Build history of the part. All positions in model axes, mm. Round coordinates to 2 decimals unless told otherwise and drop trailing zeros. Loops run counter-clockwise (first coordinate to the right, second up) from the corner with the lowest first, then second, coordinate; pieces in that order, holes last. Notation, with made-up numbers: (31, -35) - (76, -35) arc R25 cw to (76, -1) - close; hole circle Ø6 at (34.25, 53.5). An arc over 180 degrees is marked (long way). Use a Markdown table: item, result.
from build123d import *

# Parameters (mm, degrees)
SKETCH1_R           = 15
BOSS_EXTRUDE1_DEPTH = 3.175
SKETCH2_R           = 1.7
SKETCH2_R_2         = 2.65
CUT_EXTRUDE1_DEPTH  = 4.175
FILLET1_R           = 5


with BuildPart() as part:
    # Sketch1 → Boss-Extrude1 (new body)
    with BuildSketch(Plane.XY):
        Polygon((-22, 22), (22, 22), (38.014690308, -22), (38.014690308, -42), (-38.014690308, -42), (-38.014690308, -22), align=None)
        Circle(SKETCH1_R, mode=Mode.SUBTRACT)
    extrude(amount=BOSS_EXTRUDE1_DEPTH)

    # Sketch2 → Cut-Extrude1 (cut, through all)
    with BuildSketch(Plane.XY.offset(3.175)):
        with Locations((15.5, 15.5)):
            Circle(SKETCH2_R)
        with Locations((15.5, -15.5)):
            Circle(SKETCH2_R)
        with Locations((-15.5, -15.5)):
            Circle(SKETCH2_R)
        with Locations((-15.5, 15.5)):
            Circle(SKETCH2_R)
        with Locations((0, -32)):
            Circle(SKETCH2_R_2)
        with Locations((28.014690308, -32)):
            Circle(SKETCH2_R_2)
        with Locations((-28.014690308, -32)):
            Circle(SKETCH2_R_2)
    extrude(amount=-CUT_EXTRUDE1_DEPTH, mode=Mode.SUBTRACT)

    # Fillet1
    fillet1_edges = [part.edges().sort_by_distance(p)[0] for p in [
        (38.014690308, -22, 1.5875),
        (38.014690308, -42, 1.5875),
        (-38.014690308, -42, 1.5875),
        (-38.014690308, -22, 1.5875),
        (-22, 22, 1.5875),
        (22, 22, 1.5875),
    ]]
    fillet(fillet1_edges, radius=FILLET1_R)


solid = part.part
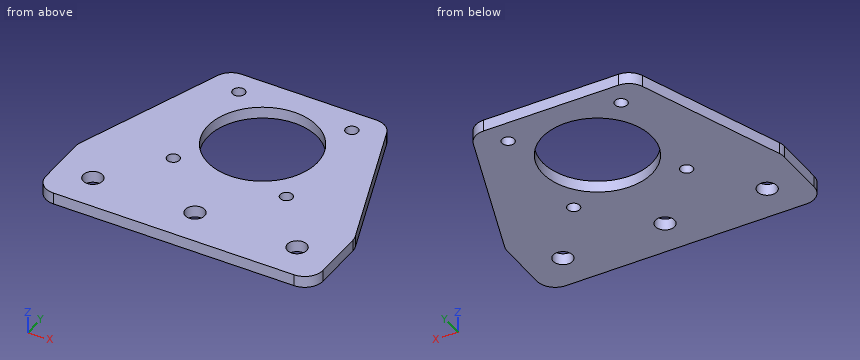
Q1. Cut at B-B, the plane y = -32. List the corners of the cut face in (x, z) (3 decimals), plus the area to 3 significant figures.
Results found:
| item | result |
|---|---|
| outline | (-38.015, 0) - (-30.665, 0) - (-30.665, 3.175) - (-38.015, 3.175) - close; (-25.365, 0) - (-2.65, 0) - (-2.65, 3.175) - (-25.365, 3.175) - close; (2.65, 0) - (25.365, 0) - (25.365, 3.175) - (2.65, 3.175) - close; (30.665, 0) - (38.015, 0) - (38.015, 3.175) - (30.665, 3.175) - close |
| area | 191 mm2 |
Q2. Cut at A-A, the plane x = -12. List the corners of the cut face in (y, z) (3 decimals).
Results found:
| item | result |
|---|---|
| outline | (-42, 0) - (-9, 0) - (-9, 3.175) - (-42, 3.175) - close; (9, 0) - (22, 0) - (22, 3.175) - (9, 3.175) - close |
Q3. Cut at C-C, the plane x = 0. List the corners of the cut face in (y, z) (3 decimals).
Results found:
| item | result |
|---|---|
| outline | (-42, 0) - (-34.65, 0) - (-34.65, 3.175) - (-42, 3.175) - close; (-29.35, 0) - (-15, 0) - (-15, 3.175) - (-29.35, 3.175) - close; (15, 0) - (22, 0) - (22, 3.175) - (15, 3.175) - close |
Q4. Probe line 1 (Y direction, x = -15.5, z = 0.7); line 2 (Y direction, x = 0, z = 1.05); line 3 (Y direction, x = -3, z = 0.5). List the from-to ranges inside material, lowest first.
Results found:
| item | result |
|---|---|
| line 1 | y = -42 to -17.2, -13.8 to 13.8, 17.2 to 22 |
| line 2 | y = -42 to -34.65, -29.35 to -15, 15 to 22 |
| line 3 | y = -42 to -14.7, 14.7 to 22 |
Q5. Cut at D-D, the plane z = 2.1. Count the separate pieces of the cut face and the enclosed holes in it, plus the area to 3 significant figures.
Results found:
| item | result |
|---|---|
| separate pieces | 1 |
| enclosed holes | 8 |
| area | 3,340 mm2 |
